```python
from build123d import *

# Parameters (mm, degrees)
SKETCH1_W                            = 76.2
SKETCH1_H                            = 21.844
STOCK_DEPTH                          = 23.749
CLEARANCE_HOLES_FOR_MOUNTING_BOLTS_D = 6.7564
SKETCH5_W                            = 76.2
SKETCH5_H                            = 4.7625
CLEARANCE_RABBIT_DEPTH               = 4.7625
SKETCH6_W                            = 11.1125
SKETCH6_H                            = 9.525
CUT_EXTRUDE1_DEPTH                   = 50.927801243


with BuildPart() as part:
    # Sketch1 → Stock (new body)
    with BuildSketch(Plane(origin=(0, 0, 0), x_dir=(1, 0, 0), z_dir=(0, 1, 0))):
        Rectangle(SKETCH1_W, SKETCH1_H)
    extrude(amount=STOCK_DEPTH)

    # Clearance holes for Mounting Bolts (through all)
    with Locations(Plane(origin=(0, 23.749, 0), x_dir=(1, 0, 0), z_dir=(0, 1, 0))):
        with Locations((-25.4, 0), (25.4, 0)):
            Hole(CLEARANCE_HOLES_FOR_MOUNTING_BOLTS_D / 2)

    # Sketch5 → Clearance Rabbit (cut)
    with BuildSketch(Plane.XZ):
        with Locations((0, 8.54075)):
            Rectangle(SKETCH5_W, SKETCH5_H)
        with Locations((0, -8.54075)):
            Rectangle(SKETCH5_W, SKETCH5_H)
    extrude(amount=-CLEARANCE_RABBIT_DEPTH, mode=Mode.SUBTRACT)

    # Sketch6 → Cut-Extrude1 (cut, through all)
    with BuildSketch(Plane.XY.offset(10.922)):
        with Locations((-25.4, 18.9865)):
            Rectangle(SKETCH6_W, SKETCH6_H)
        with Locations((25.4, 18.9865)):
            Rectangle(SKETCH6_W, SKETCH6_H)
    extrude(amount=-CUT_EXTRUDE1_DEPTH, mode=Mode.SUBTRACT)


solid = part.part
```
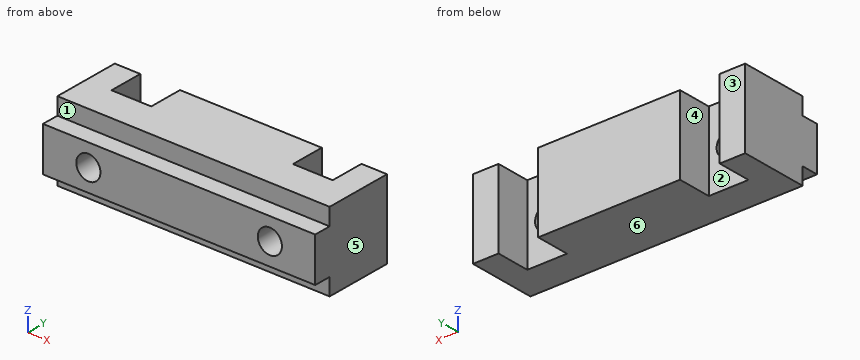
Model file for the job. Use its own axes, mm. Face numbers are marked on the shaded views. A direction names the side the tool comes from. Give positions to 0.01 mm unless a question says otherwise; leave off trailing zeros. Write each loop counter-clockwise with the first axis right and the second up, starting at its lowest first coordinate (ties: lowest second). Pieces come first, ordered by that corner, then holes. Notation, with made-up numbers: M 87,-33 L 135,-33 A26 cw 135,-9 Z; hole C 76,16 d11. An arc over 180 degrees is marked long. Use a Markdown table: item, result.
1) Pull direction X, two halves, no side cores. Call the marked faces 4, 5 and 6: +X half, -X half, draft (parallel to the pull), parting line (faces both ways), or undercut.
Responses:
| item | result |
|---|---|
| face 4 | undercut |
| face 5 | +X half |
| face 6 | draft |
2) Tool access for the marked faces 1, 2 and 3: list every direction of +Z, -Z, +X, -X, +Y, -Y with a clear straight run to the whole face (end or side of a thin tool).
Responses:
| item | result |
|---|---|
| face 1 | +Z, +X, -X, -Y |
| face 2 | +Z, -Z, +Y |
| face 3 | +Z, -Z, +X, -X, +Y |
3) Cut at B-B (z = -2.25). List the corners of the cut face in (x, y), and give its area (3 significant figures).
Responses:
| item | result |
|---|---|
| outline | M -38.1,0 L -27.92,0 L -27.92,14.22 L -30.96,14.22 L -30.96,23.75 L -38.1,23.75 Z; M -22.88,0 L 22.88,0 L 22.88,14.22 L 19.84,14.22 L 19.84,23.75 L -19.84,23.75 L -19.84,14.22 L -22.88,14.22 Z; M 27.92,0 L 38.1,0 L 38.1,23.75 L 30.96,23.75 L 30.96,14.22 L 27.92,14.22 Z |
| area | 1,450 mm2 |
4) Cut at D-D (z = -9.5). List the corners of the cut face in (x, y).
Responses:
| item | result |
|---|---|
| outline | M -38.1,4.76 L 38.1,4.76 L 38.1,23.75 L 30.96,23.75 L 30.96,14.22 L 19.84,14.22 L 19.84,23.75 L -19.84,23.75 L -19.84,14.22 L -30.96,14.22 L -30.96,23.75 L -38.1,23.75 Z |
5) Cut at A-A (y = 21.5). List the corners of the cut face in (x, z), and give its area (3 significant figures).
Responses:
| item | result |
|---|---|
| outline | M -38.1,-10.92 L -30.96,-10.92 L -30.96,10.92 L -38.1,10.92 Z; M -19.84,-10.92 L 19.84,-10.92 L 19.84,10.92 L -19.84,10.92 Z; M 30.96,-10.92 L 38.1,-10.92 L 38.1,10.92 L 30.96,10.92 Z |
| area | 1,180 mm2 |
6) Drill centre lines: line 1 (X direction, y = 18, z = -2.25); line 2 (X direction, y = 9, z = 1.75); line 3 (Z direction, x = -25.4, y = 5.5). Where is each one in solid material? Low to high. Write a range as from..to.
Responses:
| item | result |
|---|---|
| line 1 | x = -38.1..-30.96, -19.84..19.84, 30.96..38.1 |
| line 2 | x = -38.1..-28.29, -22.51..22.51, 28.29..38.1 |
| line 3 | z = -10.92..-3.38, 3.38..10.92 |
7) Pin check, flat tips, straight feed: pin 1 (1.4 mm diameter, centred on x = -16, y = 2, fed in from -Z); pin 2 (1.4 mm diameter, centred on x = -19, z = -8, fed in from -Y); pin 3 (8 mm diameter, centred on x = -25.4, z = 0, fed in from +Y). Stop position of each tip, or through.
Responses:
| item | result |
|---|---|
| pin 1 | stops at z = -6.16 |
| pin 2 | stops at y = 4.76 |
| pin 3 | stops at y = 14.22 |
8) Cut at C-C (y = 12.5). List the corners of the cut face in (x, z), and give its area (3 significant figures).
Responses:
| item | result |
|---|---|
| outline | M -38.1,-10.92 L 38.1,-10.92 L 38.1,10.92 L -38.1,10.92 Z; hole C -25.4,0 d6.76; hole C 25.4,0 d6.76 |
| area | 1,590 mm2 |
